Build history of the part. All positions in model axes, mm. Face numbers are marked on the shaded views. A direction names the side the tool comes from. Round coordinates to 2 decimals unless told otherwise and drop trailing zeros. Write each loop counter-clockwise with the first axis right and the second up, starting at its lowest first coordinate (ties: lowest second). Pieces come first, ordered by that corner, then holes.
1) Saw through at C-C (z = 9). Write the cut outline in (x, y), plus the area to 3 significant figures.
2) Saw through at B-B (y = 7.25). Write the cut outline in (x, z), plus the area to 3 significant figures.
3) Saw through at D-D (z = -14). Write the cut outline in (x, y), plus the area to 3 significant figures.
4) Saw through at A-A (x = 2.15). Write the cut outline in (y, z), plus the area to 3 significant figures.
5) Wall check: probe 1 along Y at (x, z) = (3.75, -23); probe 2 along Z at (x, y) = (2.5, 12); probe 3 along Z at (x, y) = (1.75, 13). Give the ranges that are in metal, low to high.
6) Pull direction Z, two halves, no side cores. Call the marked faces 3, 4 and 5: +Z half, -Z half, draft (parallel to the pull), parting line (faces both ways), or undercut.
7) Which spindle directions (+Z, -Z, +X, -X, +Y, -Y) get a long thin tool onto all of the face, cutting with end or side? Do the marked faces 1 and 2. Say none if no direction does.
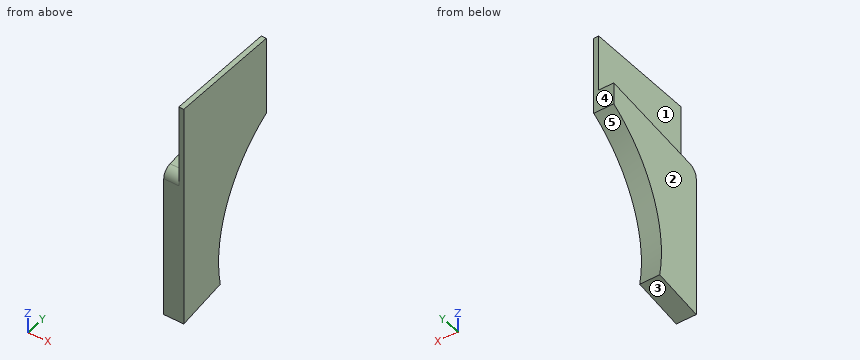
Autodesk Inventor part; units mm, degrees
ref_plane "YZ Plane" through (0, 0, 0) normal (1, 0, 0) x (0, 1, 0)
ref_plane "XZ Plane" through (0, 0, 0) normal (0, 1, 0) x (-1, 0, 0)
ref_plane "XY Plane" through (0, 0, 0) normal (0, 0, 1) x (1, 0, 0)
sketch "Sketch1" plane through (0, 0, 0) normal (1, 0, 0) x (0, 1, 0)
  line L0 (0, 0) -> (0, -30.0167)
  line L1 (0, 0) -> (22.2363, 3.4344)
  line L2 (22.2363, 3.4344) -> (22.2363, -0.9099)
  arc A0 (22.2363, -0.9099) -> (9.8481, -28.2802) centre (35.4748, -23.3905) ccw
  line L3 (0, -30.0167) -> (9.8481, -28.2802)
  dimension "d27" = 30.0167
  dimension "d28" = 22.5
  dimension "d29" = 98.78
  dimension "d35" = 9.8481
  dimension "d36" = 80
  dimension "d37" = 26.089
  dimension "d38" = 13.2384
extrude "Extrusion1" add sketch "Sketch1" along normal blind 3
fillet "Fillet2" radius 2 1 edges at (1.5, 0, 0)
sketch "Sketch3" plane through (3, 0, 0) normal (1, 0, 0) x (0, 0, -1)
  line L0 (-3.4344, 22.2363) -> (-0.2618, 1.6947)
  line L1 (-3.4344, 22.2363) -> (-14.6844, 22.2363)
  line L2 (-14.6844, 22.2363) -> (-14.6844, 0)
  line L3 (1.7148, 0) -> (30.0167, 0)
  line L4 (-14.6844, 0) -> (30.0167, 0)
  arc A0 (0.9099, 22.2363) -> (28.2802, 9.8481) centre (23.3905, 35.4748) ccw
  line L5 (-3.4344, 22.2363) -> (0.9099, 22.2363)
  arc A1 (0.9099, 22.2363) -> (28.2802, 9.8481) centre (23.3905, 35.4748) ccw
  line L6 (30.0167, 0) -> (28.2802, 9.8481)
  line L7 (28.2802, 9.8481) -> (30.0167, 0)
  point P0 (0, 0)
  dimension "d32" = 11.25
extrude "Extrusion3" add sketch "Sketch3" along normal blind 1
properties part number "jam-protector"
Evaluation:
1. outline: (3, 0) - (4, 0) - (4, 22.24) - (3, 22.24) - close
1. area: 22.2 mm2
2. outline: (0, -28.74) - (4, -28.74) - (4, 14.68) - (3, 14.68) - (3, 1.12) - (0, 1.12) - close
2. area: 133 mm2
3. outline: (0, 0) - (4, 0) - (4, 11.13) - (0, 11.13) - close
3. area: 44.5 mm2
4. outline: (0, -30.02) - (9.85, -28.28) arc R26.09 cw to (22.24, -0.91) - (22.24, 3.43) - (1.69, 0.26) arc R2 ccw to (0, -1.71) - close
4. area: 408 mm2
5. probe 1: y = 0 to 9.39
5. probe 2: z = -12.01 to 1.85
5. probe 3: z = -10.14 to 2.01
6. face 3: -Z half
6. face 4: draft
6. face 5: undercut
7. face 1: +Z, -X, -Y
7. face 2: +Z, -Z, -X, +Y, -Y
